Model file for the job. Use its own axes, mm. Face numbers are marked on the shaded views. A direction names the side the tool comes from. Coordinates: 2 decimals unless noted, no trailing zeros. Write each loop counter-clockwise with the first axis right and the second up, starting at its lowest first coordinate (ties: lowest second). Pieces come first, ordered by that corner, then holes. Notation, with made-up numbers: M -15,78.5 L 42,78.5 A32 cw 42,111.5 Z; hole C 23.25,-33 d7. An arc over 180 degrees is marked long. One line per question, with ' | ' between items. Start each with the question number.
(1) Wall check: probe 1 along Y at (x, z) = (0, 1.3) (3 decimals); probe 2 along X at (y, z) = (-9, 3.95); probe 3 along X at (y, z) = (-6.75, 1.25) (3 decimals). Give the ranges that are in metal, low to high.
(2) Tool access for the marked faces 1, 2 and 3: list every direction of +Z, -Z, +X, -X, +Y, -Y with a clear straight run to the whole face (end or side of a thin tool).
(3) Cut at D-D (x = 2.25). Write the cut outline in (y, z).
(4) Cut at B-B (y = -4.5). Write the cut outline in (x, z).
(5) Two-plate mould, pull along X, no slides. Class the marked faces 4, 5 and 6: +X half, -X half, draft (parallel to the pull), parting line (faces both ways), or undercut.
(6) Cut at A-A (z = 0.6). Write the cut outline in (x, y) (3 decimals).
(7) Flat gauge pins, fed straight in: pin 1 Ø1.5 at (x, y) = (2, -7.5) entering from +Z; pin 2 Ø3 at (x, y) = (0, 1) entering from -Z; pin 3 Ø3 at (x, y) = (0, 0) entering from -Z; pin 4 Ø1.5 at (x, z) = (-2.5, 2.5) entering from +Y. Where does each tip first touch, or does it go through?
(8) Cut at C-C (y = -0.25). Write the cut outline in (x, z), plus the area to 3 significant figures.
from build123d import *

# Parameters (mm, degrees)
ESBO_O1_R                = 1.75
RESSALTO_EXTRUS_O1_DEPTH = 4.5
ESBO_O2_R                = 2.5
ESBO_O2_R_2              = 1.75
RESSALTO_EXTRUS_O2_DEPTH = 0.5
CORTE_EXTRUS_O1_DEPTH    = 15.326548782
ESBO_O4_R                = 2.9
CORTE_EXTRUS_O2_DEPTH    = 1
ESBO_O5_R                = 2.9
CORTE_EXTRUS_O3_DEPTH    = 1.25
ESBO_O6_R                = 2.9
CORTE_EXTRUS_O4_DEPTH    = 1.5
ESBO_O7_R                = 2.9
CORTE_EXTRUS_O5_DEPTH    = 1.75
ESBO_O8_R                = 2.9
CORTE_EXTRUS_O6_DEPTH    = 2
ESBO_O9_R                = 2.9
CORTE_EXTRUS_O7_DEPTH    = 2.25
ESBO_O10_R               = 2.9
CORTE_EXTRUS_O8_DEPTH    = 3


with BuildPart() as part:
    # Esboço1 → Ressalto-extrusão1 (new body)
    with BuildSketch(Plane.XY):
        with BuildLine():
            Line((-4, 0), (-4, -9))
            ThreePointArc((-4, -9), (0, -13), (4, -9))
            Line((4, -9), (4, 0))
            ThreePointArc((4, 0), (0, 4), (-4, 0))
        make_face()
        Circle(ESBO_O1_R, mode=Mode.SUBTRACT)
    extrude(amount=RESSALTO_EXTRUS_O1_DEPTH)

    # Esboço2 → Ressalto-extrusão2 (add)
    with BuildSketch(Plane.XY.offset(4.5)):
        Circle(ESBO_O2_R)
        Circle(ESBO_O2_R_2, mode=Mode.SUBTRACT)
    extrude(amount=RESSALTO_EXTRUS_O2_DEPTH)

    # Esboço3 → Corte-extrusão1 (cut, through all)
    with BuildSketch(Plane.XY.offset(4.5)):
        with BuildLine():
            Line((-1.625, -6.5), (-1.625, -9))
            ThreePointArc((-1.625, -9), (0, -10.625), (1.625, -9))
            Line((1.625, -9), (1.625, -6.5))
            ThreePointArc((1.625, -6.5), (0, -4.875), (-1.625, -6.5))
        make_face()
    extrude(amount=-CORTE_EXTRUS_O1_DEPTH, mode=Mode.SUBTRACT)

    # Esboço4 → Corte-extrusão2 (cut)
    with BuildSketch(Plane.XY.offset(4.5)):
        with Locations((0, -9)):
            Circle(ESBO_O4_R)
    extrude(amount=-CORTE_EXTRUS_O2_DEPTH, mode=Mode.SUBTRACT)

    # Esboço5 → Corte-extrusão3 (cut)
    with BuildSketch(Plane.XY.offset(4.5)):
        with Locations((0, -8.5)):
            Circle(ESBO_O5_R)
    extrude(amount=-CORTE_EXTRUS_O3_DEPTH, mode=Mode.SUBTRACT)

    # Esboço6 → Corte-extrusão4 (cut)
    with BuildSketch(Plane.XY.offset(4.5)):
        with Locations((0, -8)):
            Circle(ESBO_O6_R)
    extrude(amount=-CORTE_EXTRUS_O4_DEPTH, mode=Mode.SUBTRACT)

    # Esboço7 → Corte-extrusão5 (cut)
    with BuildSketch(Plane.XY.offset(4.5)):
        with Locations((0, -7.5)):
            Circle(ESBO_O7_R)
    extrude(amount=-CORTE_EXTRUS_O5_DEPTH, mode=Mode.SUBTRACT)

    # Esboço8 → Corte-extrusão6 (cut)
    with BuildSketch(Plane.XY.offset(4.5)):
        with Locations((0, -7)):
            Circle(ESBO_O8_R)
    extrude(amount=-CORTE_EXTRUS_O6_DEPTH, mode=Mode.SUBTRACT)

    # Esboço9 → Corte-extrusão7 (cut)
    with BuildSketch(Plane.XY.offset(4.5)):
        with Locations((0, -6.5)):
            Circle(ESBO_O9_R)
    extrude(amount=-CORTE_EXTRUS_O7_DEPTH, mode=Mode.SUBTRACT)

    # Esboço10 → Corte-extrusão8 (cut)
    with BuildSketch(Plane(origin=(0, 0, 0), x_dir=(-1, 0, 0), z_dir=(0, 0, -1))):
        Circle(ESBO_O10_R)
    extrude(amount=-CORTE_EXTRUS_O8_DEPTH, mode=Mode.SUBTRACT)


solid = part.part
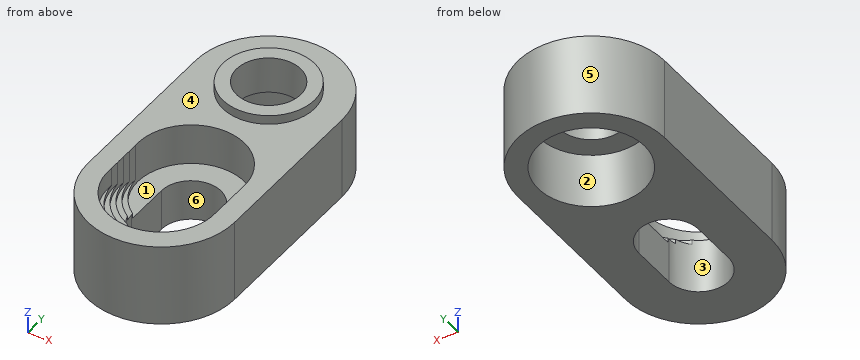
Filled in:
1) probe 1: -13 to -10.625, -4.875 to -2.9, 2.9 to 4 | probe 2: -4 to -2.9, 2.9 to 4 | probe 3: -4 to -1.625, 1.625 to 4
2) face 1: +Z | face 2: -Z | face 3: +Z, -Z
3) outline: M -12.31,0 L -1.83,0 L -1.83,3 L 1.83,3 L 1.83,0 L 3.31,0 L 3.31,4.5 L 1.09,4.5 L 1.09,5 L -1.09,5 L -1.09,4.5 L -4.67,4.5 L -4.67,2.25 L -8.33,2.25 L -8.33,2.5 L -8.83,2.5 L -8.83,2.75 L -9.33,2.75 L -9.33,3 L -9.83,3 L -9.83,3.25 L -10.33,3.25 L -10.33,3.5 L -10.83,3.5 L -10.83,4.5 L -12.31,4.5 Z
4) outline: M -4,0 L 4,0 L 4,4.5 L 2.1,4.5 L 2.1,2.25 L -2.1,2.25 L -2.1,4.5 L -4,4.5 Z
5) face 4: draft | face 5: parting line | face 6: undercut
6) outline: M -4,-9 A4 ccw 4,-9 L 4,0 A4 ccw -4,0 Z; hole C 0,0 d5.8; hole M -1.625,-9 A1.625 ccw 1.625,-9 L 1.625,-6.5 A1.625 ccw -1.625,-6.5 Z
7) pin 1: z = 2.5 | pin 2: z = 3 | pin 3: through | pin 4: y = 3.6
8) outline: M -4,0 L -2.89,0 L -2.89,3 L -1.73,3 L -1.73,5 L -2.49,5 L -2.49,4.5 L -4,4.5 Z; M 1.73,3 L 2.89,3 L 2.89,0 L 4,0 L 4,4.5 L 2.49,4.5 L 2.49,5 L 1.73,5 Z | area: 14.2 mm²
